The drawing under review shows one solid part. Ordinate dimensions are in mm from its lowest x, y, z. A direction names the side the tool comes from. Coordinates: 2 decimals unless noted, no trailing zeros. Write each loop counter-clockwise with the first axis right and the second up, starting at its lowest first coordinate (ties: lowest second). Pieces come first, ordered by that corner, then holes. Notation, with made-up numbers: (-38, 69) -> (0, 69) arc R22 cw to (0, 92) -> close; hole circle Ø5 at (-28.75, 25). An arc over 180 degrees is marked (long way). One line per item, written item: value. Start each with the question number.
1) For probe 1 along Y at (x, z) = (57.5, 28.45); probe 2 along Y at (x, z) = (50.5, 28.5); probe 3 along Z at (x, y) = (60.5, 34), list the stretches that pass through material, from the lowest coordinate up. Write a range as from..to.
2) For pin 1 Ø24 at (x, y) = (57.5, 32.5) entering from +Z, flat-tipped, find the tip position at first contact; note if it passes through.
3) Add section B-B (y = 32.5). State the section outline as (x, z) points, and give its area (3 significant figures).
4) Add section A-A (x = 57.5). State the section outline as (y, z) points.
5) Machinability: for the marked faces 1 and 2, which of the approach directions +Z, -Z, +X, -X, +Y, -Y give a long, thin tool a straight path to every point of the face, cutting with its end or side? Answer none if there is none.
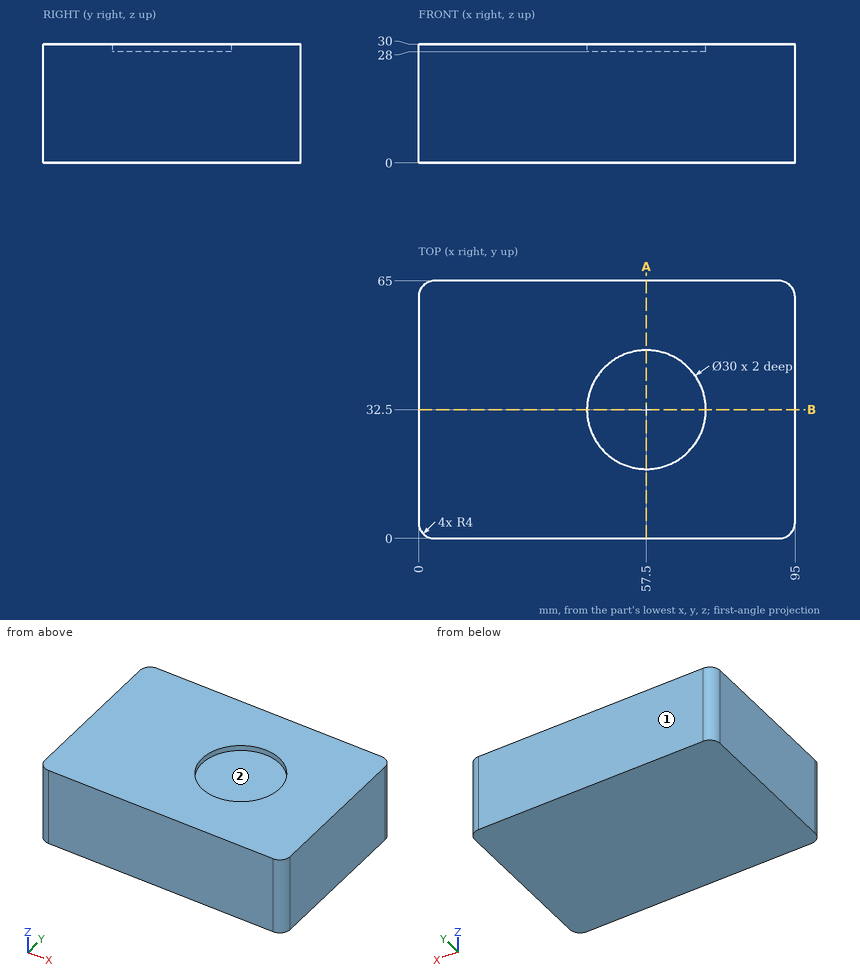
Numbers:
1. probe 1: 0..17.5, 47.5..65
1. probe 2: 0..19.23, 45.77..65
1. probe 3: 0..28
2. pin 1: z = 28
3. outline: (0, 0) -> (95, 0) -> (95, 30) -> (72.5, 30) -> (72.5, 28) -> (42.5, 28) -> (42.5, 30) -> (0, 30) -> close
3. area: 2,790 mm²
4. outline: (0, 0) -> (65, 0) -> (65, 30) -> (47.5, 30) -> (47.5, 28) -> (17.5, 28) -> (17.5, 30) -> (0, 30) -> close
5. face 1: +Z, -Z, +X, -X, +Y
5. face 2: +Z
